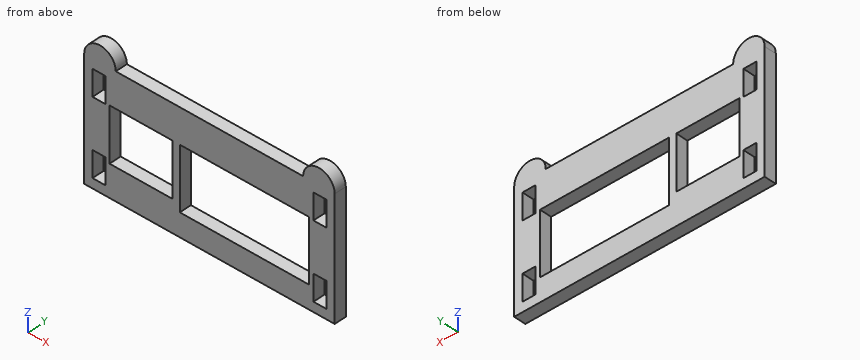
```python
from build123d import *

# Parameters (mm, degrees)
SKETCH1_W           = 3.429
SKETCH1_H           = 6.858
SKETCH1_W_2         = 34.29
SKETCH1_H_2         = 16.51
SKETCH1_W_3         = 16.764
SKETCH1_H_3         = 14.224
BOSS_EXTRUDE1_DEPTH = 3.175


with BuildPart() as part:
    # Sketch1 → Boss-Extrude1 (new body)
    with BuildSketch(Plane(origin=(0, 0, 0), x_dir=(1, 0, 0), z_dir=(0, 1, 0))):
        with BuildLine():
            Line((-24.892, -15.875), (24.892, -15.875))
            ThreePointArc((24.892, -15.875), (29.083, -20.066), (33.274, -15.875))
            Line((33.274, -15.875), (33.274, 15.875))
            Line((33.274, 15.875), (-33.274, 15.875))
            Line((-33.274, 15.875), (-33.274, -15.875))
            ThreePointArc((-33.274, -15.875), (-29.083, -20.066), (-24.892, -15.875))
        make_face()
        with Locations((29.3497, 9.906)):
            Rectangle(SKETCH1_W, SKETCH1_H, mode=Mode.SUBTRACT)
        with Locations((29.3497, -9.906)):
            Rectangle(SKETCH1_W, SKETCH1_H, mode=Mode.SUBTRACT)
        with Locations((-29.3497, -9.906)):
            Rectangle(SKETCH1_W, SKETCH1_H, mode=Mode.SUBTRACT)
        with Locations((-29.3497, 9.906)):
            Rectangle(SKETCH1_W, SKETCH1_H, mode=Mode.SUBTRACT)
        with Locations((9.271, 1.524)):
            Rectangle(SKETCH1_W_2, SKETCH1_H_2, mode=Mode.SUBTRACT)
        with Locations((-18.161, 0.381)):
            Rectangle(SKETCH1_W_3, SKETCH1_H_3, mode=Mode.SUBTRACT)
    extrude(amount=BOSS_EXTRUDE1_DEPTH)


solid = part.part
```
Here's how the part is built. I have some questions about the finished solid (model axes, mm). Coordinates: 2 decimals unless noted, no trailing zeros. Loops run counter-clockwise (first coordinate to the right, second up) from the corner with the lowest first, then second, coordinate; pieces in that order, holes last. Notation, with made-up numbers: (-23.75, -7.75) - (32.25, -7.75) arc R24 ccw to (32.25, 28.25) - close; hole circle Ø4 at (-39.75, -14.5). An arc over 180 degrees is marked (long way). Answer as CSV lines item,"result".
Q1. If we section it at C-C, the plane y = 0.65: Give the number of separate pieces and of enclosed holes in the cut face, and give its area (3 significant figures).
Response:
separate pieces,"1"
enclosed holes,"6"
area,"1,270 mm2"
Q2. If we section it at A-A, the plane z = -5: Write out the boundary of the cut face in (x, y) (3 decimals), and give its area (3 significant figures).
Response:
outline,"(-33.274, 0) - (-26.543, 0) - (-26.543, 3.175) - (-33.274, 3.175) - close; (-9.779, 0) - (-7.874, 0) - (-7.874, 3.175) - (-9.779, 3.175) - close; (26.416, 0) - (33.274, 0) - (33.274, 3.175) - (26.416, 3.175) - close"
area,"49.2 mm2"
Q3. If we section it at D-D, the plane x = -10.5: Write out the boundary of the cut face in (y, z) (3 decimals), and give its area (3 significant figures).
Response:
outline,"(0, -15.875) - (3.175, -15.875) - (3.175, -7.493) - (0, -7.493) - close; (0, 6.731) - (3.175, 6.731) - (3.175, 15.875) - (0, 15.875) - close"
area,"55.6 mm2"
Q4. For pin 1 (1 mm diameter, centred on x = -0.5, y = 2, fed in from +Z) (3 decimals), with a flat end and sliding along its axis, tell me the tip position at first contact or that it passes through.
Response:
pin 1,"z = 15.875"
Q5. If I drill on L1, parallel to X at y = 2.8, z = -11; L2, parallel to X at y = 2.8, z = -3; L3, parallel to Z at x = 29, y = 2.8 (3 decimals), over which ranges is the centre line in solid material (lowest first)? Write a range as [from, to].
Response:
L1,"[-33.27, -31.06], [-27.64, 27.64], [31.06, 33.27]"
L2,"[-33.27, -26.54], [-9.78, -7.87], [26.42, 33.27]"
L3,"[-15.875, -13.335], [-6.477, 6.477], [13.335, 20.065]"
Q6. If we section it at B-B, the plane x = 14: Write out the boundary of the cut face in (y, z) (3 decimals), and give its area (3 significant figures).
Response:
outline,"(0, -15.875) - (3.175, -15.875) - (3.175, -9.779) - (0, -9.779) - close; (0, 6.731) - (3.175, 6.731) - (3.175, 15.875) - (0, 15.875) - close"
area,"48.4 mm2"
